Geometry check sheet. Reference: drawing and pictorial views, mm from the part's lowest x, y, z. A direction names the side the tool comes from. Give positions to 0.01 mm unless a question says otherwise; leave off trailing zeros. Write each loop counter-clockwise with the first axis right and the second up, starting at its lowest first coordinate (ties: lowest second). Pieces come first, ordered by that corner, then holes. Notation, with made-up numbers: M 5,-15 L 49,-15 A18 cw 49,2 Z; hole C 40.25,-28.5 d6. An arc over 180 degrees is marked long. One line per item, written item: value. Start each with the question number.
1. Tool access check on the marked faces 1, 2 and 3. Record the directions out of +Z, -Z, +X, -X, +Y, -Y that give a thin tool (end or side, any length) a straight path to the whole face; none if there is none.
2. Cross-section at D-D on z = 38. Record the cut outline in (x, y).
3. Cross-section at A-A on y = 11. Record the cut outline in (x, z), then the cut area to 3 significant figures.
4. Scan lines: line 1 (Y direction, x = 122.5, z = 99); line 2 (Z direction, x = 108, y = 5); line 3 (X direction, y = 7.5, z = 71.5). Record each from-to range of solid material in increasing order.
5. Cross-section at B-B on x = 147.5. Record the cut outline in (y, z), then the cut area to 3 significant figures.
6. Gauge pin test, flat ends, axial feed: pin 1 (19 mm diameter, centred on x = 139.5, z = 64.5, fed in from -Y); pin 2 (7.5 mm diameter, centred on x = 136, y = 13.5, fed in from +Z); pin 3 (12 mm diameter, centred on y = 16.5, z = 76.5, fed in from +X). Record the tip position at first contact, or that the pin passes through.
7. Cross-section at C-C on z = 92. Record the cut outline in (x, y), then the cut area to 3 significant figures.
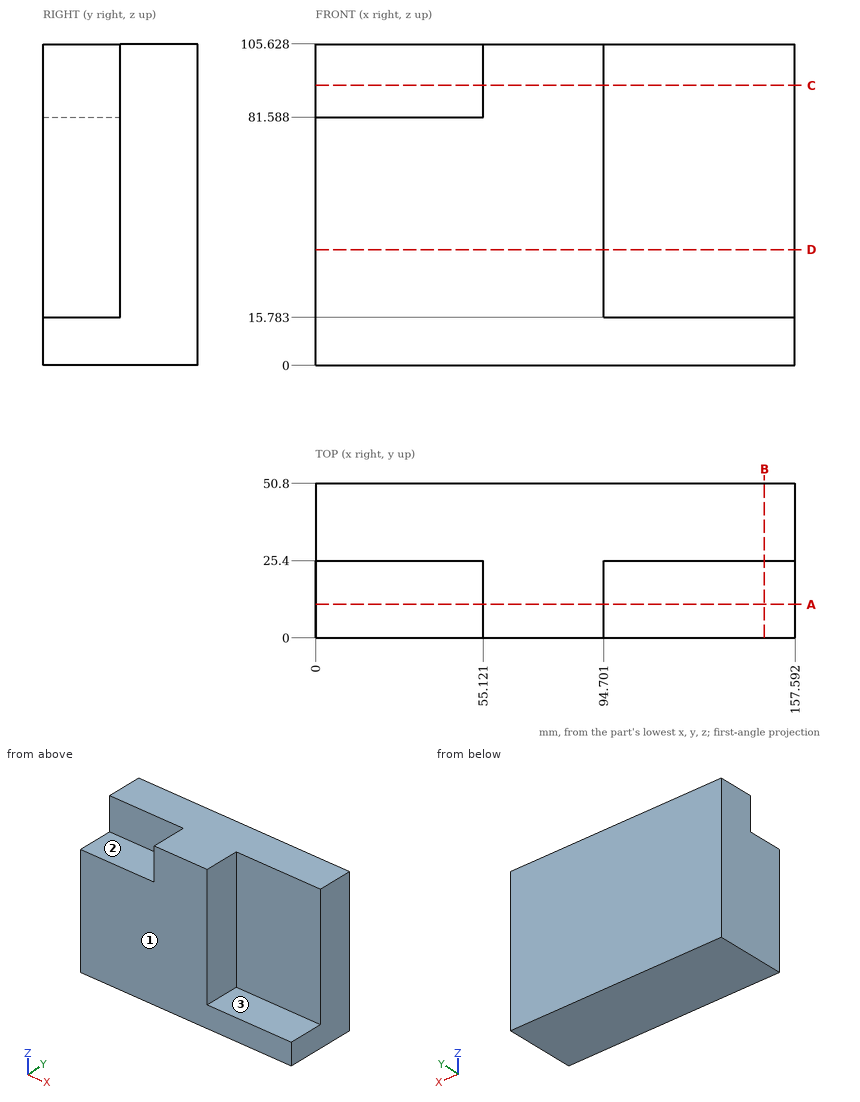
Report:
1. face 1: +Z, -Z, +X, -X, -Y
1. face 2: +Z, -X, -Y
1. face 3: +Z, +X, -Y
2. outline: M 0,0 L 94.7,0 L 94.7,25.4 L 157.59,25.4 L 157.59,50.8 L 0,50.8 Z
3. outline: M 0,0 L 157.59,0 L 157.59,15.78 L 94.7,15.78 L 94.7,105.63 L 55.12,105.63 L 55.12,81.59 L 0,81.59 Z
3. area: 9,670 mm^2
4. line 1: y = 25.4 to 50.8
4. line 2: z = 0 to 15.78
4. line 3: x = 0 to 94.7
5. outline: M 0,0 L 50.8,0 L 50.8,105.63 L 25.4,105.63 L 25.4,15.78 L 0,15.78 Z
5. area: 3,080 mm^2
6. pin 1: stops at y = 25.4
6. pin 2: stops at z = 15.78
6. pin 3: stops at x = 94.7
7. outline: M 0,25.4 L 55.12,25.4 L 55.12,0 L 94.7,0 L 94.7,25.4 L 157.59,25.4 L 157.59,50.8 L 0,50.8 Z
7. area: 5,010 mm^2
